Read the model definition and answer for the solid it produces. Units are mm, in the model's axes. Face numbers are marked on the shaded views. A direction names the side the tool comes from. Give positions to 0.01 mm unless a question says otherwise; leave off trailing zeros. Write each loop counter-clockwise with the first axis right and the second up, starting at its lowest first coordinate (ties: lowest second). Pieces come first, ordered by that corner, then holes.
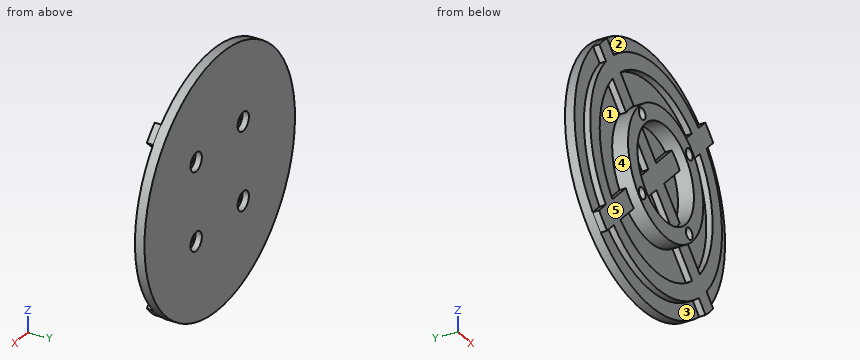
```python
from build123d import *

# Parameters (mm, degrees)
SKETCH_1_R               = 40
EXTRUDE_1_DEPTH          = 3
SKETCH_2_R               = 35
SKETCH_2_R_2             = 30
EXTRUDE_2_DEPTH          = 2
SKETCH_3_R               = 20
SKETCH_3_R_2             = 15
EXTRUDE_3_DEPTH          = 5
EXTRUDE_START            = 2
EXTRUDE_5_DEPTH          = 2
EXTRUDE_4_DEPTH          = 2
CUT_EXTRUDE_2_DEPTH      = 57.789083458
CUT_EXTRUDE_2_DEPTH_BACK = 57.789083458
SKETCH_8_R               = 1.8
CUT_EXTRUDE_3_DEPTH      = 58.131427428
CUT_EXTRUDE_3_DEPTH_BACK = 2
SKETCH_9_R               = 3


with BuildPart() as part:
    # 草图1 → 凸台-拉伸1 (new body)
    with BuildSketch(Plane(origin=(0, 0, 0), x_dir=(1, 0, 0), z_dir=(0, 1, 0))):
        with Locations(Location((0, 0, 0), (0, 0, 270))):
            Circle(SKETCH_1_R)
    extrude(amount=EXTRUDE_1_DEPTH)

    # 草图2 → 凸台-拉伸2 (add)
    with BuildSketch(Plane.XZ):
        with Locations(Location((0, 0, 0), (0, 0, 90))):
            Circle(SKETCH_2_R)
        with Locations(Location((0, 0, 0), (0, 0, 270))):
            Circle(SKETCH_2_R_2, mode=Mode.SUBTRACT)
    extrude(amount=EXTRUDE_2_DEPTH)

    # 草图3 → 凸台-拉伸3 (add)
    with BuildSketch(Plane.XZ):
        with Locations(Location((0, 0, 0), (0, 0, 90))):
            Circle(SKETCH_3_R)
        with Locations(Location((0, 0, 0), (0, 0, 270))):
            Circle(SKETCH_3_R_2, mode=Mode.SUBTRACT)
    extrude(amount=EXTRUDE_3_DEPTH)

    # 草图7 → 凸台-拉伸5 (add)
    with BuildSketch(Plane.XZ.offset(EXTRUDE_START)):
        with BuildLine():
            Line((-26.083289209, 30.325929896), (30.325929896, -26.083289209))
            ThreePointArc((30.325929896, -26.083289209), (28.356463256, -28.211894506), (26.237952221, -30.192215275))
            Line((26.237952221, -30.192215275), (-30.192215275, 26.237952221))
            ThreePointArc((-30.192215275, 26.237952221), (-28.211894506, 28.356463256), (-26.083289209, 30.325929896))
        make_face()
    extrude(amount=-EXTRUDE_5_DEPTH)

    # 草图6 → 凸台-拉伸4 (add)
    with BuildSketch(Plane.XZ.offset(EXTRUDE_START)):
        with BuildLine():
            Line((-30.327162218, -26.081856372), (26.087002686, 30.322735543))
            ThreePointArc((26.087002686, 30.322735543), (28.286671146, 28.281871146), (30.327162218, 26.081856372))
            Line((30.327162218, 26.081856372), (-26.087002686, -30.322735543))
            ThreePointArc((-26.087002686, -30.322735543), (-28.286671146, -28.281871146), (-30.327162218, -26.081856372))
        make_face()
    extrude(amount=-EXTRUDE_4_DEPTH)

    # 草图8 → 切除-拉伸2 (cut, two sides: drawn at the far end of the back side and taken through both)
    with BuildSketch(Plane.XZ.offset(-CUT_EXTRUDE_2_DEPTH_BACK)):
        with Locations(Location((12.5, -12.5, 0), (0, 0, 270))):
            Circle(SKETCH_8_R)
        with Locations(Location((12.5, 12.5, 0), (0, 0, 270))):
            Circle(SKETCH_8_R)
        with Locations(Location((-12.5, -12.5, 0), (0, 0, 270))):
            Circle(SKETCH_8_R)
        with Locations(Location((-12.5, 12.5, 0), (0, 0, 270))):
            Circle(SKETCH_8_R)
    extrude(amount=CUT_EXTRUDE_2_DEPTH + CUT_EXTRUDE_2_DEPTH_BACK, mode=Mode.SUBTRACT)

    # 草图9 → 切除-拉伸3 (cut, two sides: drawn at the far end of the back side and taken through both)
    with BuildSketch(Plane(origin=(0, 3, 0), x_dir=(1, 0, 0), z_dir=(0, 1, 0)).offset(-CUT_EXTRUDE_3_DEPTH_BACK)):
        with Locations(Location((-12.5, 12.5, 0), (0, 0, 90))):
            Circle(SKETCH_9_R)
        with Locations(Location((12.5, 12.5, 0), (0, 0, 90))):
            Circle(SKETCH_9_R)
        with Locations(Location((-12.5, -12.5, 0), (0, 0, 90))):
            Circle(SKETCH_9_R)
        with Locations(Location((12.5, -12.5, 0), (0, 0, 90))):
            Circle(SKETCH_9_R)
    extrude(amount=CUT_EXTRUDE_3_DEPTH + CUT_EXTRUDE_3_DEPTH_BACK, mode=Mode.SUBTRACT)


solid = part.part
```
Item 1: Which of the six approach directions +Z, -Z, +X, -X, +Y, -Y give full straight-line access (tool end or side, diameter ignored) to the marked faces 1, 2 and 3?
Result set:
face 1: -Y
face 2: +Z, -Y
face 3: -Z, -Y
Item 2: Find the intervals of material crossed by line 1 along X through (y, z) = (-1.75, -12.5); line 2 along Z through (x, y) = (-16.5, -0.5); line 3 along X through (y, z) = (2.25, 12), in increasing order.
Result set:
line 1: x = -32.69 to -27.27, -16.74 to -14.3, -10.7 to -8.26, 8.29 to 10.7, 14.3 to 16.74, 27.27 to 32.69
line 2: z = -30.87 to -25.05, -20.74 to -12.26, -11.3 to 11.3, 12.55 to 20.74, 25.05 to 30.87
line 3: x = -38.16 to -15.46, -9.54 to 9.54, 15.46 to 38.16
Item 3: Determine the mould class of the marked faces 4 and 5 for opening direction Z: pulls with the +Z half, pulls with the -Z half, needs draft (parallel to the pull), parting line crosses it, or undercut.
Result set:
face 4: undercut
face 5: needs draft
Item 4: Each of these flat-tipped pins is pushed along its axis until it touches: pin 1 Ø3 at (x, z) = (-12.5, -12.5) entering from -Y; pin 2 Ø8.5 at (x, z) = (-8.5, -2) entering from -Y; pin 3 Ø3 at (x, z) = (0, -11) entering from -Y; pin 4 Ø4 at (y, z) = (-0.5, 25) entering from -X. Where does it stop, or does it pass through?
Result set:
pin 1: passes through
pin 2: stops at y = -2
pin 3: stops at y = 0
pin 4: stops at x = -32.68
Item 5: Section C-C (x = -1) is taken. Write down the section's boundary in (y, z), and give its area (3 significant figures).
Result set:
outline: (-5, -19.97) - (0, -19.97) - (0, -29.98) - (-2, -29.98) - (-2, -34.99) - (0, -34.99) - (0, -39.99) - (3, -39.99) - (3, 39.99) - (0, 39.99) - (0, 34.99) - (-2, 34.99) - (-2, 29.98) - (0, 29.98) - (0, 19.97) - (-5, 19.97) - (-5, 14.97) - (0, 14.97) - (0, 5.24) - (-2, 5.24) - (-2, -5.24) - (0, -5.24) - (0, -14.97) - (-5, -14.97) - close
area: 331 mm2
Item 6: Section A-A (y = -4) is taken. Write down the section's boundary in (x, z), and give its area (3 significant figures).
Result set:
outline: circle Ø40 at (0, 0); hole circle Ø30 at (0, 0); hole circle Ø3.6 at (-12.5, -12.5); hole circle Ø3.6 at (-12.5, 12.5); hole circle Ø3.6 at (12.5, -12.5); hole circle Ø3.6 at (12.5, 12.5)
area: 509 mm2
Item 7: Section B-B (x = -34) is taken. Write down the section's boundary in (y, z), and give its area (3 significant figures).
Result set:
outline: (-2, -8.31) - (0, -8.31) - (0, -21.07) - (3, -21.07) - (3, 21.07) - (0, 21.07) - (0, 8.31) - (-2, 8.31) - close
area: 160 mm2
